```python
from build123d import *

# Parameters (mm, degrees)
F0_R     = 317.5
F1_DEPTH = 12.7
F2_DEPTH = 1.5875
F3_R     = 12.69999


# Not quite as in the source:
# - a fillet or chamfer is up to 0.001 mm smaller than in the source, because OpenCascade refuses the exact size


with BuildPart() as f1:
    # F0 (on Front) → F1 (new body, symmetric)
    with BuildSketch(Plane.XZ):
        Circle(F0_R)
        with BuildLine():
            ThreePointArc((207.6362893124, 205.4497051849), (269.4299975889, 112.8267982318), (292.075151117, 3.81))
            ThreePointArc((292.075151117, 3.81), (292.0937877132, 1.9050405158), (292.1, 0))
            ThreePointArc((292.1, 0), (292.0937877132, -1.9050405158), (292.075151117, -3.81))
            ThreePointArc((292.075151117, -3.81), (274.1141878064, -100.9149247795), (224.8232220619, -186.4857335607))
            ThreePointArc((224.8232220619, -186.4857335607), (222.371673788, -189.4023460697), (219.8822912949, -192.2867337465))
            ThreePointArc((219.8822912949, -192.2867337465), (122.4703733828, -265.1856286519), (3.81, -292.075151117))
            ThreePointArc((3.81, -292.075151117), (0, -292.1), (-3.81, -292.075151117))
            ThreePointArc((-3.81, -292.075151117), (-110.7351842209, -270.2963724795), (-202.2065364328, -210.7959359756))
            ThreePointArc((-202.2065364328, -210.7959359756), (-204.9388469754, -208.1405270493), (-207.6362893124, -205.4497051849))
            ThreePointArc((-207.6362893124, -205.4497051849), (-269.4299975889, -112.8267982318), (-292.075151117, -3.81))
            ThreePointArc((-292.075151117, -3.81), (-292.1, 0), (-292.075151117, 3.81))
            ThreePointArc((-292.075151117, 3.81), (-274.1141878064, 100.9149247795), (-224.8232220619, 186.4857335607))
            ThreePointArc((-224.8232220619, 186.4857335607), (-222.371673788, 189.4023460697), (-219.8822912949, 192.2867337465))
            ThreePointArc((-219.8822912949, 192.2867337465), (-122.4703733828, 265.1856286519), (-3.81, 292.075151117))
            ThreePointArc((-3.81, 292.075151117), (0, 292.1), (3.81, 292.075151117))
            ThreePointArc((3.81, 292.075151117), (110.7351842209, 270.2963724795), (202.2065364328, 210.7959359756))
            ThreePointArc((202.2065364328, 210.7959359756), (204.9388469754, 208.1405270493), (207.6362893124, 205.4497051849))
        make_face(mode=Mode.SUBTRACT)
    extrude(amount=F1_DEPTH, both=True)

    # F0 (on Front) → F2 (join, symmetric)
    with BuildSketch(Plane.XZ):
        with BuildLine():
            ThreePointArc((-3.81, 12.115027858), (0, 12.7), (3.81, 12.115027858))
            Line((3.81, 12.115027858), (3.81, 292.075151117))
            ThreePointArc((3.81, 292.075151117), (0, 292.1), (-3.81, 292.075151117))
            Line((-3.81, 292.075151117), (-3.81, 12.115027858))
        make_face()
        with BuildLine():
            ThreePointArc((-11.6934678579, 4.9550791574), (-9.668333643, 8.2348846117), (-6.7525370909, 10.7560793432))
            Line((-6.7525370909, 10.7560793432), (-219.8822912949, 192.2867337465))
            ThreePointArc((-219.8822912949, 192.2867337465), (-222.371673788, 189.4023460697), (-224.8232220619, 186.4857335607))
            Line((-224.8232220619, 186.4857335607), (-11.6934678579, 4.9550791574))
        make_face()
        with BuildLine():
            ThreePointArc((5.7850887786, 11.3058722717), (8.9103846511, 9.0495881326), (11.2148416582, 5.959641481))
            Line((11.2148416582, 5.959641481), (207.6362893124, 205.4497051849))
            ThreePointArc((207.6362893124, 205.4497051849), (204.9388469754, 208.1405270493), (202.2065364328, 210.7959359756))
            Line((202.2065364328, 210.7959359756), (5.7850887786, 11.3058722717))
        make_face()
        with BuildLine():
            ThreePointArc((12.115027858, 3.81), (12.5529051179, 1.9273227809), (12.7, 0))
            ThreePointArc((12.7, 0), (12.5529051179, -1.9273227809), (12.115027858, -3.81))
            Line((12.115027858, -3.81), (292.075151117, -3.81))
            ThreePointArc((292.075151117, -3.81), (292.0937877132, -1.9050405158), (292.1, 0))
            ThreePointArc((292.1, 0), (292.0937877132, 1.9050405158), (292.075151117, 3.81))
            Line((292.075151117, 3.81), (12.115027858, 3.81))
        make_face()
        with BuildLine():
            Line((224.8232220619, -186.4857335607), (11.6934678579, -4.9550791574))
            ThreePointArc((11.6934678579, -4.9550791574), (9.668333643, -8.2348846117), (6.7525370909, -10.7560793432))
            Line((6.7525370909, -10.7560793432), (219.8822912949, -192.2867337465))
            ThreePointArc((219.8822912949, -192.2867337465), (222.371673788, -189.4023460697), (224.8232220619, -186.4857335607))
        make_face()
        with BuildLine():
            Line((3.81, -292.075151117), (3.81, -12.115027858))
            ThreePointArc((3.81, -12.115027858), (0, -12.7), (-3.81, -12.115027858))
            Line((-3.81, -12.115027858), (-3.81, -292.075151117))
            ThreePointArc((-3.81, -292.075151117), (0, -292.1), (3.81, -292.075151117))
        make_face()
        with BuildLine():
            ThreePointArc((-12.115027858, -3.81), (-12.7, 0), (-12.115027858, 3.81))
            Line((-12.115027858, 3.81), (-292.075151117, 3.81))
            ThreePointArc((-292.075151117, 3.81), (-292.1, 0), (-292.075151117, -3.81))
            Line((-292.075151117, -3.81), (-12.115027858, -3.81))
        make_face()
        with BuildLine():
            Line((-202.2065364328, -210.7959359756), (-5.7850887786, -11.3058722717))
            ThreePointArc((-5.7850887786, -11.3058722717), (-8.9103846511, -9.0495881326), (-11.2148416582, -5.959641481))
            Line((-11.2148416582, -5.959641481), (-207.6362893124, -205.4497051849))
            ThreePointArc((-207.6362893124, -205.4497051849), (-204.9388469754, -208.1405270493), (-202.2065364328, -210.7959359756))
        make_face()
        with BuildLine():
            ThreePointArc((12.115027858, -3.81), (12.5529051179, -1.9273227809), (12.7, 0))
            ThreePointArc((12.7, 0), (12.5529051179, 1.9273227809), (12.115027858, 3.81))
            ThreePointArc((12.115027858, 3.81), (11.7143477213, 4.9055129666), (11.2148416582, 5.959641481))
            ThreePointArc((11.2148416582, 5.959641481), (8.9103846511, 9.0495881326), (5.7850887786, 11.3058722717))
            ThreePointArc((5.7850887786, 11.3058722717), (4.814573227, 11.7520161948), (3.81, 12.115027858))
            ThreePointArc((3.81, 12.115027858), (0, 12.7), (-3.81, 12.115027858))
            ThreePointArc((-3.81, 12.115027858), (-5.3247988427, 11.5298099414), (-6.7525370909, 10.7560793432))
            ThreePointArc((-6.7525370909, 10.7560793432), (-9.668333643, 8.2348846117), (-11.6934678579, 4.9550791574))
            ThreePointArc((-11.6934678579, 4.9550791574), (-11.9180081655, 4.3876054252), (-12.115027858, 3.81))
            ThreePointArc((-12.115027858, 3.81), (-12.7, 0), (-12.115027858, -3.81))
            ThreePointArc((-12.115027858, -3.81), (-11.7143477213, -4.9055129666), (-11.2148416582, -5.959641481))
            ThreePointArc((-11.2148416582, -5.959641481), (-8.9103846511, -9.0495881326), (-5.7850887786, -11.3058722717))
            ThreePointArc((-5.7850887786, -11.3058722717), (-4.814573227, -11.7520161948), (-3.81, -12.115027858))
            ThreePointArc((-3.81, -12.115027858), (0, -12.7), (3.81, -12.115027858))
            ThreePointArc((3.81, -12.115027858), (5.3247988427, -11.5298099414), (6.7525370909, -10.7560793432))
            ThreePointArc((6.7525370909, -10.7560793432), (9.668333643, -8.2348846117), (11.6934678579, -4.9550791574))
            ThreePointArc((11.6934678579, -4.9550791574), (11.9180081655, -4.3876054252), (12.115027858, -3.81))
        make_face()
    extrude(amount=F2_DEPTH, both=True)

    # F3 (radius 12.7 in the source; OpenCascade refuses exactly that, so slightly less here)
    f3_edges = [f1.edges().sort_by_distance(p)[0] for p in [
        (-317.5, -12.7, 0),
        (-317.5, 12.7, 0),
    ]]
    fillet(f3_edges, radius=F3_R)


solid = f1.part
```
Geometry: final body of the model. Coordinates: model frame, mm. A direction names the side the tool comes from. Round coordinates to 2 decimals unless told otherwise and drop trailing zeros. Order: outer loops, then holes, each group sorted by start corner. A loop starts at its lowest first (then second) coordinate and runs counter-clockwise, first axis right, second up. Notation, with made-up numbers: (54.25, 72.25) -> (58.25, 72.25) arc R8 cw to (58.25, 78.25) -> close; hole circle Ø5 at (3.25, -23). An arc over 180 degrees is marked (long way). Write each question's results on one line, items separated by ' | '.
Q1. Access query for faces 1 (the face through (-108.05, -0.02, -104.31)), 2 (the face through (-1, -1.588, 1)), 3 (the face through (247, -12.7, -157)), 4 (the face through (-1, 1.588, 1)). Directions: +Z, -Z, +X, -X, +Y, -Y. A direction counts if a zero-diameter tool reaches every point of the face in a straight line with its end or side. Return the directions, or none.
Response values:
face 1: +Y, -Y | face 2: -Y | face 3: +Z, -Z, +X, -X, -Y | face 4: +Y
Q2. Ray query, line 1 along X through (y, z) = (-1.5, 184); line 2 along X through (y, z) = (-0.5, -19); line 3 along Y through (x, z) = (-170.5, -174). Return the intervals inside material, ascending.
Response values:
line 1: -258.64 to -226.86, -221.9 to -210.15, -3.81 to 3.81, 175.82 to 186.52, 226.86 to 258.64 | line 2: -316.92 to -291.48, -24.05 to -13.36, -3.81 to 3.81, 16.43 to 28.18, 291.48 to 316.92 | line 3: -1.59 to 1.59
Q3. Section query B-B (x = 141). Count the separate pieces of the cut face and the enclosed holes in it, and give its area (3 significant figures).
Response values:
separate pieces: 5 | enclosed holes: 0 | area: 1,390 mm²
Q4. Section query A-A (y = 6.25). Output: boundary loops of the cut face in (x, z), and give its area (3 significant figures).
Response values:
outline: circle Ø631.71 at (0, 0); hole circle Ø584.2 at (0, 0) | area: 45,400 mm²
Q5. Pull-direction query (Z, two-part tool) for faces 5 (the face through (105.371, -0.022, 112.447)), 6 (the face through (247, 12.7, -157)), 7 (the face through (119.75, -0.02, -96.99)); classes: released by +Z, released by -Z, zero draft, split by the parting line, or undercut.
Response values:
face 5: undercut | face 6: zero draft | face 7: undercut
Q6. Pin query (flat end, axial travel): pin 1 Ø2.5 at (x, y) = (149.5, 0) entering from +Z; pin 2 Ø8 at (x, y) = (208, -10) entering from -Z; pin 3 Ø10 at (y, z) = (-9.5, -100.5) entering from -X. Return the tip coordinate at first contact, or that it passes through.
Response values:
pin 1: z = 280.76 | pin 2: z = -239.39 | pin 3: x = -300.85
